The model under review builds one solid part; all positions refer to its coordinate system, in mm. A direction names the side the tool comes from. Give positions to 0.01 mm unless a question says otherwise; leave off trailing zeros. Write each loop counter-clockwise with the first axis right and the second up, starting at its lowest first coordinate (ties: lowest second). Pieces come first, ordered by that corner, then holes. Notation, with made-up numbers: (5.5, 65) - (35.5, 65) arc R19 cw to (35.5, 76) - close; hole circle Ø11 at (78.25, -13). An arc over 180 degrees is marked (long way). Write item = value, one per line.
```python
from build123d import *

# Parameters (mm, degrees)
F1_DEPTH = 25.4
F3_DEPTH = 7.62


with BuildPart() as f1:
    # F0 (on Top) → F1 (new body)
    with BuildSketch(Plane.XY):
        with BuildLine():
            Line((-21.94954, -30.042156), (0, -65.198988))
            Line((0, -65.198988), (21.94954, -30.042156))
            Line((21.94954, -30.042156), (30.500225, -8.054676))
            Line((30.500225, -8.054676), (30.500225, 34.393379))
            Line((30.500225, 34.393379), (21.94954, 52.410898))
            Line((21.94954, 52.410898), (4.490128, 69.87031))
            ThreePointArc((4.490128, 69.87031), (0, 71.730182), (-4.490128, 69.87031))
            Line((-4.490128, 69.87031), (-21.94954, 52.410898))
            Line((-21.94954, 52.410898), (-30.500225, 34.393379))
            Line((-30.500225, 34.393379), (-30.500225, -8.054676))
            Line((-30.500225, -8.054676), (-21.94954, -30.042156))
        make_face()
        Polygon((-15.445927, 52.410898), (-4.490128, 63.366696), (0, 65.380182), (4.490128, 63.366696), (15.445927, 52.410898), (23.996611, 34.393379), (23.996611, -8.054676), (15.445927, -30.042156), (0, -54.782075), (-15.445927, -30.042156), (-23.996611, -8.054676), (-23.996611, 34.393379), align=None, mode=Mode.SUBTRACT)
    extrude(amount=F1_DEPTH)

    # F2 (on Top) → F3 (join)
    with BuildSketch(Plane.XY):
        Polygon((-16.171693, 53.127095), (-23.972463, 34.050059), (-23.972463, -7.481851), (-15.727157, -29.774714), (0, -54.20525), (15.727157, -29.774714), (23.667078, -8.092615), (23.667078, 33.744678), (15.727157, 52.067574), (5.649563, 62.45055), (0, 66.115133), (-6.565708, 62.45055), align=None)
    extrude(amount=F3_DEPTH)


solid = f1.part
```
1. Take a section at C-C on z = 17. Give the boundary of the cut face in (x, y).
Findings below:
outline = (-30.5, -8.05) - (-21.95, -30.04) - (0, -65.2) - (21.95, -30.04) - (30.5, -8.05) - (30.5, 34.39) - (21.95, 52.41) - (4.49, 69.87) arc R6.35 ccw to (-4.49, 69.87) - (-21.95, 52.41) - (-30.5, 34.39) - close; hole (-24, -8.05) - (-15.45, -30.04) - (0, -54.78) - (15.45, -30.04) - (24, -8.05) - (24, 34.39) - (15.45, 52.41) - (4.49, 63.37) - (0, 65.38) - (-4.49, 63.37) - (-15.45, 52.41) - (-24, 34.39) - close
2. Draft analysis for pull direction X (two halves, no side actions). For faces 4 (the flat face through (-26.165, 43.528, 12.522)), 5 (the cylindrical face through (0.07, 71.73, 12.52)), 6 (the flat face through (19.781, -18.895, 12.522)), state which applies: +X half, -X half, draft (parallel to the pull), parting line (faces both ways), or undercut.
Findings below:
face_4 = -X half
face_5 = parting line
face_6 = undercut
3. Take a section at B-B on z = 5.25. Count the separate pieces of the cut face and the enclosed holes in it, and give its area (3 significant figures).
Findings below:
separate_pieces = 1
enclosed_holes = 5
area = 5,900 mm²
4. Take a section at D-D on x = -2. Give the boundary of the cut face in (y, z), and give its area (3 significant figures).
Findings below:
outline = (-62, 0) - (-51.58, 0) - (-51.58, 25.4) - (-62, 25.4) - close; (-51.1, 0) - (71.41, 0) - (71.41, 25.4) - (64.48, 25.4) - (64.48, 7.62) - (-51.1, 7.62) - close
area = 1,320 mm²
5. Machinability: for faces 1 (the flat face through (26.165, -19.202, 12.522)), 2 (the flat face through (23.667, 13, 4)), 3 (the flat face through (0, 6, 7.62)), which of the approach directions +Z, -Z, +X, -X, +Y, -Y give a long, thin tool a straight path to every point of the face, cutting with its end or side? Answer none if there is none.
Findings below:
face_1 = +Z, -Z, +X, -Y
face_2 = +Z, -Z
face_3 = +Z
6. Take a section at A-A on y = -2. Give the boundary of the cut face in (x, z).
Findings below:
outline = (-30.5, 0) - (-24, 0) - (-24, 25.4) - (-30.5, 25.4) - close; (-23.97, 0) - (23.67, 0) - (23.67, 7.62) - (-23.97, 7.62) - close; (24, 0) - (30.5, 0) - (30.5, 25.4) - (24, 25.4) - close
7. Insertion check: P1, Ø5, axis at x = -18.5, z = 16, coming from the +Y side; P2, Ø12, axis at x = 19, y = -12.5, coming from the +Z side; P3, Ø2, axis at x = 0, y = 43, coming from the +Z side; P4, Ø4, axis at y = -15.5, z = 5, coming from the +X side. Each pin has a flat end and moves straight along its axis. Give the tip position at first contact, or say it passes through.
Findings below:
P1 = 58.36
P2 = 25.4
P3 = 7.62
P4 = 28.38
8. For line 1 (X direction, y = 13, z = 18); line 2 (Z direction, x = -11, y = 45.5); line 3 (X direction, y = -38, z = 15.75), list the stretches that pass through material, from the lowest coordinate up. Write a range as from..to.
Findings below:
line_1 = -30.5..-24, 24..30.5
line_2 = 0..7.62
line_3 = -16.98..-10.48, 10.48..16.98
